Build history of the part. All positions in model axes, mm. Face numbers are marked on the shaded views. A direction names the side the tool comes from. Give positions to 0.01 mm unless a question says otherwise; leave off trailing zeros. Write each loop counter-clockwise with the first axis right and the second up, starting at its lowest first coordinate (ties: lowest second). Pieces come first, ordered by that corner, then holes. Notation, with made-up numbers: M -39,84 L 5,84 A16 cw 5,106 Z; hole C 61,87.5 d6. An arc over 180 degrees is marked long. Return JSON: item names as keys, results as strings. Group by question number.
Q1. Band-saw the part on A-A, the plane x = 14. Give the cut face in (y, z).
Q2. Wall check: probe 1 along Y at (x, z) = (12, 3.5); probe 2 along Z at (x, y) = (7, 46.5); probe 3 along X at (y, z) = (32, -19) (3 decimals). Give the ranges that are in metal, low to high.
Q3. Band-saw the part on B-B, the plane z = -8.5. Give the cut face in (x, y) (3 decimals).
Q4. Band-saw the part on C-C, the plane y = 45. Give the cut face in (x, z) (3 decimals), then the cut area to 3 significant figures.
Q5. Band-saw the part on D-D, the plane z = 14. Give the cut face in (x, y) (3 decimals).
Q6. Pull direction X, two halves, no side cores. Call the marked faces 1, 2, 3 and 4: +X half, -X half, draft (parallel to the pull), parting line (faces both ways), or undercut.
Q7. Tool access for the marked faces 5 and 6: list every direction of +Z, -Z, +X, -X, +Y, -Y with a clear straight run to the whole face (end or side of a thin tool).
Q8. Flat gauge pins, fed straight in: pin 1 Ø6 at (x, y) = (18.5, 50.5) entering from +Z; pin 2 Ø1 at (x, z) = (12.5, 15.5) entering from +Y; pin 3 Ø1.5 at (x, z) = (5, -6.5) entering from +Y. Where does each tip first touch, or does it go through?
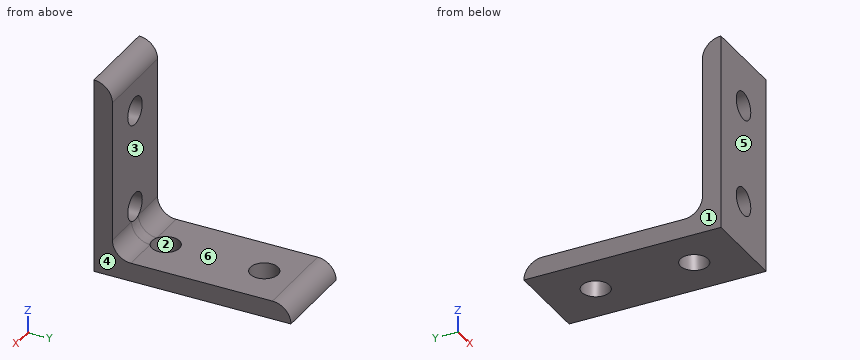
from build123d import *

# Parameters (mm, degrees)
EXTRUDE1_DEPTH     = 22.225
SKETCH2_R          = 3.5687
CUT_EXTRUDE1_DEPTH = 5.7752
FILLET1_R          = 4.7752


with BuildPart() as part:
    # Sketch1 → Extrude1 (new body)
    with BuildSketch(Plane(origin=(0, 0, 0), x_dir=(0, 0, -1), z_dir=(1, 0, 0))):
        with BuildLine():
            Line((-28.199163803, 21.897674685), (22.600836197, 21.897674685))
            Line((22.600836197, 21.897674685), (17.825636197, 26.672874685))
            Line((17.825636197, 26.672874685), (-23.423963803, 26.672874685))
            ThreePointArc((-23.423963803, 26.672874685), (-26.800540105, 25.274250987), (-28.199163803, 21.897674685))
        make_face()
    extrude(amount=EXTRUDE1_DEPTH)

    # Sketch2 → Cut-Extrude1 (cut, through all)
    with BuildSketch(Plane(origin=(0, 26.672874685, 0), x_dir=(1, 0, 0), z_dir=(0, 1, 0))):
        with Locations((11.1125, -15.499163803)):
            Circle(SKETCH2_R)
        with Locations((11.1125, 9.900836197)):
            Circle(SKETCH2_R)
    extrude(amount=-CUT_EXTRUDE1_DEPTH, mode=Mode.SUBTRACT)

    # Mirror1: part across plane


with BuildPart() as part_1:
    add(part.part)
    add(part.part.mirror(Plane(origin=(22.225, 21.897674685, -22.600836197), x_dir=(0, 0.707106781, 0.707106781), z_dir=(0, -0.707106781, 0.707106781))))

    # Fillet1
    fillet1_edges = [part_1.edges().sort_by_distance(p)[0] for p in [
        (11.1125, 26.672874685, -17.825636197),
    ]]
    fillet(fillet1_edges, radius=FILLET1_R)


solid = part_1.part
From the geometry:
{
 "1": {"outline": "M 21.9,-22.6 L 32.5,-22.6 L 32.5,-17.83 L 31.45,-17.83 A4.78 cw 26.67,-13.05 L 26.67,-12 L 21.9,-12 Z; M 21.9,-7.8 L 26.67,-7.8 L 26.67,13.4 L 21.9,13.4 Z; M 21.9,17.6 L 26.67,17.6 L 26.67,23.42 A4.78 ccw 21.9,28.2 Z; M 36.69,-22.6 L 57.9,-22.6 L 57.9,-17.83 L 36.69,-17.83 Z; M 62.09,-22.6 L 72.7,-22.6 A4.78 ccw 67.92,-17.83 L 62.09,-17.83 Z"},
 "2": {"probe 1": "y = 21.9 to 26.67", "probe 2": "z = -22.6 to -17.83", "probe 3": "x = 0 to 8.666, 13.559 to 22.225"},
 "3": {"outline": "M 0,21.898 L 7.83,21.898 L 7.83,26.673 L 0,26.673 Z; M 14.395,21.898 L 22.225,21.898 L 22.225,26.673 L 14.395,26.673 Z"},
 "4": {"outline": "M 0,-22.601 L 22.225,-22.601 L 22.225,-17.826 L 0,-17.826 Z", "area": "106 mm^2"},
 "5": {"outline": "M 0,21.898 L 7.874,21.898 L 7.874,26.673 L 0,26.673 Z; M 14.351,21.898 L 22.225,21.898 L 22.225,26.673 L 14.351,26.673 Z"},
 "6": {"face 1": "-X half", "face 2": "undercut", "face 3": "draft", "face 4": "+X half"},
 "7": {"face 5": "+Z, -Z, +X, -X, -Y", "face 6": "+Z, +X, -X, +Y"},
 "8": {"pin 1": "stops at z = -17.83", "pin 2": "passes through", "pin 3": "stops at y = 26.67"}
}
